Here's how the part is built. I have some questions about the finished solid (model axes, mm). A direction names the side the tool comes from. Coordinates: 2 decimals unless noted, no trailing zeros. Write each loop counter-clockwise with the first axis right and the second up, starting at its lowest first coordinate (ties: lowest second). Pieces come first, ordered by that corner, then holes.
Item 1: If we section it at D-D (z = -2.75): Please give me the cut outline in (x, y), then the cut area to 3 significant figures.
Item 2: If I drill on line 1 (X direction, y = -0.25, z = 1); line 2 (Y direction, x = 0, z = 1.5); line 3 (X direction, y = 1.5, z = 4), over which ranges is the centre line in solid material (lowest first)?
Item 3: If we section it at B-B (z = 0): Please give me the cut outline in (x, y), then the cut area to 3 significant figures.
Item 4: For faces 1 (the face through (-0.75, -11, -1)), 2 (the face through (5, -11, -2)), 3 (the face through (7.982, -0.448, -0.064)), which set-ups out of +Z, -Z, +X, -X, +Y, -Y let a thin tool reach every point of the face, with its end or its side?
Item 5: I'm going to push flat-ended pins straight in: pin 1 Ø5 at (y, z) = (-9, 0) entering from -X; pin 2 Ø3.5 at (x, y) = (0, 10) entering from +Z; pin 3 Ø1.5 at (x, y) = (-2, 4) entering from +Z; pin 4 Ø1 at (x, z) = (7, -0.5) entering from -Y. Where does each tip first touch, or does it pass through?
Item 6: If we section it at A-A (y = 0): Count the separate pieces of the cut face and the enclosed holes in it, then the cut area to 3 significant figures.
Item 7: We'd pull the mould along X, two halves only. Please class faces 4 (the face through (0.634, 14.629, -4.858)), 5 (the face through (-12.018, -0.448, -0.064)), 6 (the face through (2.9, -6.77, 0.29)): +X half, -X half, draft (parallel to the pull), parting line (faces both ways), or undercut.
Autodesk Inventor part; units mm, degrees
ref_plane "to_bolt_XY" through (5, -9, 0) normal (1, 0, 0) x (0, 0, -1)
ref_plane "to_bolt_YZ" through (5, -9, 0) normal (0, 0, -1) x (0, 1, 0)
ref_plane "to_bolt_ZX" through (5, -9, 0) normal (0, 1, 0) x (1, 0, 0)
sketch "Sketch_14" plane through (0, 0, 0) normal (1, 0, 0) x (0, 1, 0)
  line L0 (0, -5) -> (0, 5)
  line L1 (0, 5) -> (14.5, 5)
  line L2 (14.5, 5) -> (15, 4.5)
  line L3 (15, 4.5) -> (15, -4.5)
  line L4 (15, -4.5) -> (14.5, -5)
  line L5 (14.5, -5) -> (0, -5)
  line L6 (0, -5) -> (0, 5)
revolve "Revolution1" add sketch "Sketch_14" angle 360 about axis through (0, 0, -5) along (0, 0, -1)
sketch "Sketch_15" plane through (0, 0, 0) normal (1, 0, 0) x (0, 1, 0)
  line L0 (0, -5) -> (0, 5)
  line L1 (0, 5) -> (5.5, 5)
  line L2 (5.5, 5) -> (5, 4.5)
  line L3 (5, 4.5) -> (5, -4.5)
  line L4 (5, -4.5) -> (5.5, -5)
  line L5 (5.5, -5) -> (0, -5)
  line L6 (0, -5) -> (0, 5)
revolve "Revolution2" cut sketch "Sketch_15" angle 360 about axis through (0, 0, -5) along (0, 0, -1)
sketch "Sketch_16" plane through (0, 0, 0) normal (0, 0, 1) x (1, 0, 0)
  arc A0 (-0.75, -15.9824) -> (0.75, -15.9824) centre (0, 0) ccw
  line L0 (0.75, -15.9824) -> (0.75, 0)
  line L1 (0.75, 0) -> (-0.75, 0)
  line L2 (-0.75, 0) -> (-0.75, -15.9824)
extrude "Extrusion1" cut sketch "Sketch_16" along normal mid plane 10
sketch "Sketch_18" plane through (10, 0, 0) normal (1, 0, 0) x (0, 0, -1)
  line L0 (5, 0) -> (-5, 0)
  line L1 (-5, 0) -> (-5, 2.5)
  line L2 (-5, 2.5) -> (-4.567, 2.067)
  line L3 (-4.567, 2.067) -> (4.567, 2.067)
  line L4 (4.567, 2.067) -> (5, 2.5)
  line L5 (5, 2.5) -> (5, 0)
  line L6 (5, 0) -> (-5, 0)
revolve "Revolution3" cut sketch "Sketch_18" angle 360 about axis through (10, 0, -5) along (0, 0, -1)
thread "Thread1"
sketch "Sketch_20" plane through (-10, 0, 0) normal (1, 0, 0) x (0, 0, -1)
  line L0 (5, 0) -> (-5, 0)
  line L1 (-5, 0) -> (-5, 2.5)
  line L2 (-5, 2.5) -> (-4.567, 2.067)
  line L3 (-4.567, 2.067) -> (4.567, 2.067)
  line L4 (4.567, 2.067) -> (5, 2.5)
  line L5 (5, 2.5) -> (5, 0)
  line L6 (5, 0) -> (-5, 0)
revolve "Revolution4" cut sketch "Sketch_20" angle 360 about axis through (-10, 0, -5) along (0, 0, -1)
thread "Thread2"
sketch "Sketch_22" plane through (0, 10, 0) normal (0, 1, 0) x (1, 0, 0)
  line L0 (0, 5) -> (0, -5)
  line L1 (0, -5) -> (-2.5, -5)
  line L2 (-2.5, -5) -> (-2.067, -4.567)
  line L3 (-2.067, -4.567) -> (-2.067, 4.567)
  line L4 (-2.067, 4.567) -> (-2.5, 5)
  line L5 (-2.5, 5) -> (0, 5)
  line L6 (0, 5) -> (0, -5)
revolve "Revolution5" cut sketch "Sketch_22" angle 360 about axis through (0, 10, -5) along (0, 0, -1)
thread "Thread3"
sketch "Sketch_23" plane through (0, -9, 0) normal (0, 1, 0) x (1, 0, 0)
  line L0 (15, 0) -> (0, 0)
  line L1 (0, 0) -> (0, 2.25)
  line L2 (0, 2.25) -> (5, 2.25)
  line L3 (5, 2.25) -> (5, 3.75)
  line L4 (5, 3.75) -> (15, 3.75)
  line L5 (15, 3.75) -> (15, 0)
  line L6 (15, 0) -> (0, 0)
revolve "Revolution6" cut sketch "Sketch_23" angle 360 about axis through (15, -9, 0) along (1, 0, 0)
sketch "Sketch_25" plane through (0, 0, 0) normal (0, 0, 1) x (1, 0, 0)
  line L0 (-0.75, -9) -> (-13.2665, -9)
  line L1 (-13.2665, -9) -> (-13.2665, -7.379)
  line L2 (-13.2665, -7.379) -> (-1.129, -7.379)
  line L3 (-1.129, -7.379) -> (-0.75, -7)
  line L4 (-0.75, -7) -> (-0.75, -9)
  line L5 (-0.75, -9) -> (-13.2665, -9)
revolve "Revolution7" cut sketch "Sketch_25" angle 360 about axis through (-0.75, -9, 0) along (1, 0, 0)
thread "Thread4"
ref_plane "to_bolt_XY" through (5, -9, 0) normal (1, 0, 0) x (0, 0, -1)
ref_plane "to_bolt_YZ" through (5, -9, 0) normal (0, 0, -1) x (0, 1, 0)
ref_plane "to_bolt_ZX" through (5, -9, 0) normal (0, 1, 0) x (1, 0, 0)
properties part number "SCSTR10-10b" material "鋼、炭素鋼"
Answer list:
1. outline: (-0.75, -14.98) - (-0.75, -4.94) arc R5 cw (long way) to (0.75, -4.94) - (0.75, -14.98) arc R15 ccw to (9.57, -11.55) - (5, -11.55) - (5, -6.45) - (13.54, -6.45) arc R15 ccw (long way) to start; hole circle Ø4.13 at (-10, 0); hole circle Ø4.13 at (0, 10); hole circle Ø4.13 at (10, 0)
1. area: 538 mm2
2. line 1: x = -15 to -12.05, -7.95 to -4.99, 4.99 to 7.95, 12.05 to 15
2. line 2: y = 5 to 7.93, 12.07 to 15
2. line 3: x = -14.92 to -11.42, -8.58 to -4.77, 4.77 to 8.58, 11.42 to 14.92
3. outline: (-13.06, -7.38) - (-1.13, -7.38) - (-0.75, -7) - (-0.75, -4.94) arc R5 cw (long way) to (0.75, -4.94) - (0.75, -6.75) - (5, -6.75) - (5, -5.25) - (14.05, -5.25) arc R15 ccw (long way) to start; (-10.59, -10.62) arc R15 ccw to (-0.75, -14.98) - (-0.75, -11) - (-1.13, -10.62) - close; (0.75, -14.98) arc R15 ccw to (7.9, -12.75) - (5, -12.75) - (5, -11.25) - (0.75, -11.25) - close; hole circle Ø4.13 at (-10, 0); hole circle Ø4.13 at (0, 10); hole circle Ø4.13 at (10, 0)
3. area: 467 mm2
4. face 1: +Z, -Z, -Y
4. face 2: +X
4. face 3: +Z, -Z
5. pin 1: stops at x = -13.52
5. pin 2: passes through
5. pin 3: stops at z = 4.72
5. pin 4: stops at y = -13.52
6. separate pieces: 4
6. enclosed holes: 0
6. area: 116 mm2
7. face 4: parting line
7. face 5: undercut
7. face 6: draft
